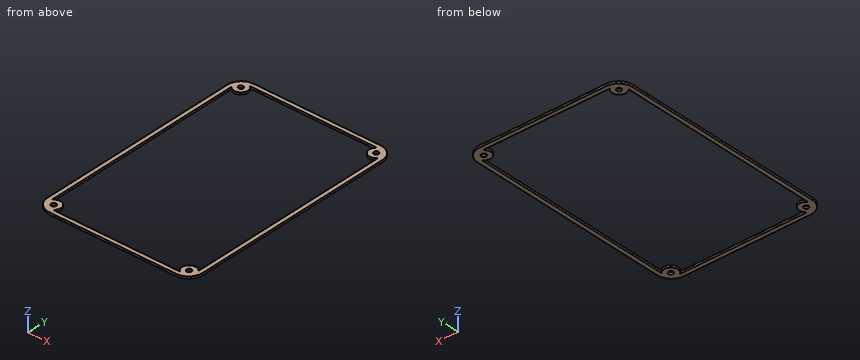
from build123d import *

# Parameters (mm, degrees)
BOSS_EXTRUDE1_DEPTH = 1.5
SKETCH2_R           = 5
BOSS_EXTRUDE2_DEPTH = 1.5
SKETCH3_R           = 1.7
CUT_EXTRUDE1_DEPTH  = 100.164005567


with BuildPart() as part:
    # Sketch1 → Boss-Extrude1 (new body)
    with BuildSketch(Plane.XY):
        with BuildLine():
            Line((-45, -82.5), (45, -82.5))
            ThreePointArc((45, -82.5), (52.071067812, -79.571067812), (55, -72.5))
            Line((55, -72.5), (55, 72.5))
            ThreePointArc((55, 72.5), (52.071067812, 79.571067812), (45, 82.5))
            Line((45, 82.5), (-45, 82.5))
            ThreePointArc((-45, 82.5), (-52.071067812, 79.571067812), (-55, 72.5))
            Line((-55, 72.5), (-55, -72.5))
            ThreePointArc((-55, -72.5), (-52.071067812, -79.571067812), (-45, -82.5))
        make_face()
        with BuildLine():
            Line((-45, -79.5), (45, -79.5))
            ThreePointArc((45, -79.5), (49.949747468, -77.449747468), (52, -72.5))
            Line((52, -72.5), (52, 72.5))
            ThreePointArc((52, 72.5), (49.949747468, 77.449747468), (45, 79.5))
            Line((45, 79.5), (-45, 79.5))
            ThreePointArc((-45, 79.5), (-49.949747468, 77.449747468), (-52, 72.5))
            Line((-52, 72.5), (-52, -72.5))
            ThreePointArc((-52, -72.5), (-49.949747468, -77.449747468), (-45, -79.5))
        make_face(mode=Mode.SUBTRACT)
    extrude(amount=BOSS_EXTRUDE1_DEPTH)

    # Sketch2 → Boss-Extrude2 (add)
    with BuildSketch(Plane.XY):
        with Locations((-48, -75.5)):
            Circle(SKETCH2_R)
        with Locations((-48, 75.5)):
            Circle(SKETCH2_R)
        with Locations((48, -75.5)):
            Circle(SKETCH2_R)
        with Locations((48, 75.5)):
            Circle(SKETCH2_R)
    extrude(amount=BOSS_EXTRUDE2_DEPTH)

    # Sketch3 → Cut-Extrude1 (cut, through all)
    with BuildSketch(Plane.XY.offset(1.5)):
        with Locations((-48, -75.5)):
            Circle(SKETCH3_R)
        with Locations((-48, 75.5)):
            Circle(SKETCH3_R)
        with Locations((48, -75.5)):
            Circle(SKETCH3_R)
        with Locations((48, 75.5)):
            Circle(SKETCH3_R)
    extrude(amount=-CUT_EXTRUDE1_DEPTH, mode=Mode.SUBTRACT)


solid = part.part
For this review, take the finished solid that the model builds, in its own axes (mm). Round coordinates to 2 decimals unless told otherwise and drop trailing zeros. Order: outer loops, then holes, each group sorted by start corner. A loop starts at its lowest first (then second) coordinate and runs counter-clockwise, first axis right, second up. Notation, with made-up numbers: M 76,-19 L 117,-19 A12 ccw 117,-15 Z; hole C 58,-25.75 d3. An arc over 180 degrees is marked long. Use a Markdown table: item, result. Add a question column.
Item 1: Add section C-C, the plane x = 26. Give the boundary of the cut face in (y, z), then the cut area to 3 significant figures.
Item 2: Add section B-B, the plane z = 0.55. Give the boundary of the cut face in (x, y), then the cut area to 3 significant figures.
Item 3: To check wall thickness, follow line 1 along X through (y, z) = (32, 0.35); line 2 along Y through (x, z) = (-42.5, 1.45); line 3 along X through (y, z) = (-75.5, 0.5). State the ranges of each line that lie inside material, in increasing order.
Item 4: Add section D-D, the plane x = -48. Give the boundary of the cut face in (y, z).
Item 5: Add section A-A, the plane y = 62. Give the boundary of the cut face in (x, z), then the cut area to 3 significant figures.
Geometry results:
| question | item | result |
|---|---|---|
| 1 | outline | M -82.5,0 L -79.5,0 L -79.5,1.5 L -82.5,1.5 Z; M 79.5,0 L 82.5,0 L 82.5,1.5 L 79.5,1.5 Z |
| 1 | area | 9.00 mm² |
| 2 | outline | M -55,-72.5 A10 ccw -45,-82.5 L 45,-82.5 A10 ccw 55,-72.5 L 55,72.5 A10 ccw 45,82.5 L -45,82.5 A10 ccw -55,72.5 Z; hole M -52,-72.5 A5 cw long -45,-79.5 L 45,-79.5 A5 cw long 52,-72.5 L 52,72.5 A5 cw long 45,79.5 L -45,79.5 A5 cw long -52,72.5 Z; hole C -48,-75.5 d3.4; hole C -48,75.5 d3.4; hole C 48,-75.5 d3.4; hole C 48,75.5 d3.4 |
| 2 | area | 1,780 mm² |
| 3 | line 1 | x = -55 to -52, 52 to 55 |
| 3 | line 2 | y = -82.5 to -79.5, 79.5 to 82.5 |
| 3 | line 3 | x = -54.54 to -49.7, -46.3 to -43, 43 to 46.3, 49.7 to 54.54 |
| 4 | outline | M -82.04,0 L -77.2,0 L -77.2,1.5 L -82.04,1.5 Z; M -73.8,0 L -70.5,0 L -70.5,1.5 L -73.8,1.5 Z; M 70.5,0 L 73.8,0 L 73.8,1.5 L 70.5,1.5 Z; M 77.2,0 L 82.04,0 L 82.04,1.5 L 77.2,1.5 Z |
| 5 | outline | M -55,0 L -52,0 L -52,1.5 L -55,1.5 Z; M 52,0 L 55,0 L 55,1.5 L 52,1.5 Z |
| 5 | area | 9.00 mm² |
